```python
from build123d import *


with BuildPart() as f2:
    # F0 (on Front) → F2 (revolve)
    with BuildSketch(Plane.XZ):
        Polygon((18.415, 84.724767), (15.875, 84.724767), (15.875, -93.075233), (18.415, -93.075233), (18.415, -36.09307), (17.145, -34.82307), (18.415, -33.55307), (18.415, -23.39307), (17.145, -22.12307), (18.415, -20.85307), (18.415, -10.69307), (17.145, -9.42307), (18.415, -8.15307), (18.415, 2.00693), (17.145, 3.27693), (18.415, 4.54693), (18.415, 14.70693), (17.145, 15.97693), (18.415, 17.24693), (18.415, 27.40693), (17.145, 28.67693), (18.415, 29.94693), (18.415, 40.10693), (17.145, 41.37693), (18.415, 42.64693), (18.415, 52.80693), (17.145, 54.07693), (18.415, 55.34693), (18.415, 65.50693), (17.145, 66.77693), (18.415, 68.04693), (18.415, 78.20693), (17.145, 79.47693), (18.415, 80.74693), align=None)
    revolve(axis=Axis((0, 0, -4.614733), (0, 0, -1)))


solid = f2.part
```
Verification items for the finished model (mm, model axes). Give positions to 0.01 mm unless a question says otherwise; leave off trailing zeros. Order: outer loops, then holes, each group sorted by start corner. A loop starts at its lowest first (then second) coordinate and runs counter-clockwise, first axis right, second up. Notation, with made-up numbers: (40.5, 73) -> (97.5, 73) arc R26 ccw to (97.5, 112) -> close; hole circle Ø7 at (2.25, 39). An arc over 180 degrees is marked (long way). Use a Markdown table: item, result.
1) Material ranges on probe 1 along Y at (x, z) = (0, 44) (3 decimals); probe 2 along Y at (x, z) = (0, 16) (3 decimals), recorded low to high.
Results:
| item | result |
|---|---|
| probe 1 | -18.415 to -15.875, 15.875 to 18.415 |
| probe 2 | -17.168 to -15.875, 15.875 to 17.168 |
2) Section check A-A, the plane z = 11. Record the boundary of the cut face in (x, y) (3 decimals), then the cut area to 3 significant figures.
Results:
| item | result |
|---|---|
| outline | circle Ø36.83 at (0, 0); hole circle Ø31.75 at (0, 0) |
| area | 274 mm² |
3) Mould release check, pull along X, two halves, no side actions. Record for faces 1 (the cylindrical face through (-14.61, 11.21, 60.5)), 2 (the cylindrical face through (-3.441, 15.497, -5.42)): pulls with the +X half, pulls with the -X half, needs draft (parallel to the pull), parting line crosses it, or undercut.
Results:
| item | result |
|---|---|
| face 1 | parting line crosses it |
| face 2 | undercut |
4) Depth check by flat-ended pin: pin 1 Ø10 at (y, z) = (8.5, 60.5) entering from +X; pin 2 Ø6 at (y, z) = (12, -60) entering from -X; pin 3 Ø3 at (x, z) = (0, -28.5) entering from -Y (3 decimals). Enter the tip coordinate at first touch or a pass-through.
Results:
| item | result |
|---|---|
| pin 1 | x = 18.08 |
| pin 2 | x = -16.07 |
| pin 3 | y = -18.415 |
